from build123d import *

# Parameters (mm, degrees)
SKETCH_1_W          = 101.5
SKETCH_1_H          = 91.5
SKETCH_1_W_2        = 98.5
SKETCH_1_H_2        = 88.5
EXTRUDE_1_DEPTH     = 21
SKETCH_2_W          = 101.5
SKETCH_2_H          = 91.5
SKETCH_2_R          = 8.25
SKETCH_2_R_2        = 6
EXTRUDE_2_DEPTH     = 1.8
SKETCH_3_R          = 1.75
CUT_EXTRUDE_1_DEPTH = 139.25881527
SKETCH_4_R          = 1.75
CUT_EXTRUDE_2_DEPTH = 139.25881527
FILLET_1_R          = 9
FILLET_2_R          = 10
FILLET_3_R          = 4
FILLET_4_R          = 5
CUT_EXTRUDE_3_DEPTH = 1
CUT_EXTRUDE_4_REACH = 140.259
SKETCH_6_R          = 5.25


with BuildPart() as part:
    # 草图1 → 凸台-拉伸1 (new body)
    with BuildSketch(Plane(origin=(0, 0, 0), x_dir=(0, 0, -1), z_dir=(1, 0, 0))):
        with Locations((50.75, 45.75)):
            Rectangle(SKETCH_1_W, SKETCH_1_H)
        with Locations((50.75, 45.75)):
            Rectangle(SKETCH_1_W_2, SKETCH_1_H_2, mode=Mode.SUBTRACT)
    extrude(amount=EXTRUDE_1_DEPTH)

    # 草图2 → 凸台-拉伸2 (add)
    with BuildSketch(Plane.ZY):
        with Locations((-50.75, 45.75)):
            Rectangle(SKETCH_2_W, SKETCH_2_H)
        with Locations((-86.5, 76.5)):
            Circle(SKETCH_2_R, mode=Mode.SUBTRACT)
        with Locations((-50.75, 43.5)):
            Circle(SKETCH_2_R_2, mode=Mode.SUBTRACT)
    extrude(amount=EXTRUDE_2_DEPTH)

    # 草图3 → 切除-拉伸1 (cut, through all)
    with BuildSketch(Plane.XY):
        with Locations((11, 45.75)):
            Circle(SKETCH_3_R)
    extrude(amount=-CUT_EXTRUDE_1_DEPTH, mode=Mode.SUBTRACT)

    # 草图4 → 切除-拉伸2 (cut, through all)
    with BuildSketch(Plane(origin=(0, 91.5, 0), x_dir=(1, 0, 0), z_dir=(0, 1, 0))):
        with Locations(Location((11, 16.75, 0), (0, 0, 270))):
            Circle(SKETCH_4_R)
        with Locations(Location((11, 84.75, 0), (0, 0, 90))):
            Circle(SKETCH_4_R)
    extrude(amount=-CUT_EXTRUDE_2_DEPTH, mode=Mode.SUBTRACT)

    # 圆角1
    fillet_1_edges = [part.edges().sort_by_distance(p)[0] for p in [
        (10.5, 90, -100),
        (10.5, 90, -1.5),
    ]]
    fillet(fillet_1_edges, radius=FILLET_1_R)

    # 圆角2
    fillet_2_edges = [part.edges().sort_by_distance(p)[0] for p in [
        (9.6, 91.5, 0),
        (9.6, 91.5, -101.5),
    ]]
    fillet(fillet_2_edges, radius=FILLET_2_R)

    # 圆角3
    fillet_3_edges = [part.edges().sort_by_distance(p)[0] for p in [
        (10.5, 1.5, -1.5),
        (10.5, 1.5, -100),
    ]]
    fillet(fillet_3_edges, radius=FILLET_3_R)

    # 圆角4
    fillet_4_edges = [part.edges().sort_by_distance(p)[0] for p in [
        (9.6, 0, -101.5),
        (9.6, 0, 0),
    ]]
    fillet(fillet_4_edges, radius=FILLET_4_R)

    # 草图5 → 切除-拉伸3 (cut)
    with BuildSketch(Plane.ZY.offset(1.8)):
        with BuildLine():
            Line((-30.75, 43.5), (-20.75, 43.5))
            ThreePointArc((-20.75, 43.5), (-45.75, 68.5), (-70.75, 43.5))
            ThreePointArc((-70.75, 43.5), (-50.75, 63.5), (-30.75, 43.5))
        make_face()
    extrude(amount=-CUT_EXTRUDE_3_DEPTH, mode=Mode.SUBTRACT)

    # 草图6 → 切除-拉伸4 (cut, up to next)
    with BuildSketch(Plane.XY, mode=Mode.PRIVATE) as cut_extrude_4_sk1:
        with Locations((9, 74.75)):
            Circle(SKETCH_6_R)
    cut_extrude_4_tool1 = extrude(cut_extrude_4_sk1.sketch, amount=-CUT_EXTRUDE_4_REACH, mode=Mode.PRIVATE) & part.part
    add(cut_extrude_4_tool1.solids().sort_by_distance((9, 74.75, 0))[0], mode=Mode.SUBTRACT)


solid = part.part
Could you check a few things on this model? Use its own coordinates, in mm. A direction names the side the tool comes from. Give positions to 0.01 mm unless a question says otherwise; leave off trailing zeros. Write each loop counter-clockwise with the first axis right and the second up, starting at its lowest first coordinate (ties: lowest second). Pieces come first, ordered by that corner, then holes. Notation, with made-up numbers: (2.5, -33) -> (29.5, -33) arc R23 cw to (29.5, 5) -> close; hole circle Ø4 at (-6.5, 36). An arc over 180 degrees is marked (long way). Answer as CSV lines item,"result". Start each with the question number.
(1) Which directions (+Z, -Z, +X, -X, +Y, -Y) give clear straight access to the entire face, cutting with the end or side of a thin tool? Please do faces 1 (the face through (-0.8, 57.9, -36.6)), 2 (the face through (10.647, 87.294, -97.434)), 3 (the face through (12.18, 0.76, -18.04)).
(2) Please list where these lines run through material, in increasing order: line 1 (Y direction, x = 15.5, z = -54.5); line 2 (Z direction, x = 6.5, y = 41.5); line 3 (Y direction, x = -1.2, z = -86.5).
(3) If we section it at A-A, the plane z = -16.75: Write out the boundary of the cut face in (x, y), and give its area (3 significant figures).
(4) If we section it at C-C, the plane y = 45.75: Give the number of separate pieces and of enclosed holes in the cut face, and give its area (3 significant figures).
(5) I'm going to push flat-ended pins straight in: pin 1 Ø3 at (x, z) = (11, -84.75) entering from +Y; pin 2 Ø4 at (y, z) = (44.5, -82.5) entering from +X. Where does each tip first touch, or does it pass through?
(6) If we section it at B-B, the plane x = 18.25: Write out the boundary of the cut face in (y, z).
(7) If we mould it in two halves opening along Y, with no side actions, what happens to faces 4 (the face through (10, 43, -1.5)), 5 (the face through (-1.307, 68.494, -45.2)), 6 (the face through (12.18, 90.76, -18.04)), 7 (the face through (9.76, 88.65, -98.49))? For each: +Y half, -Y half, draft (parallel to the pull), parting line (faces both ways), or undercut.
(8) If we section it at D-D, the plane y = 33.5: Write out the boundary of the cut face in (x, z), and give its area (3 significant figures).
Answer list:
1,face 1,"-X"
1,face 2,"+X"
1,face 3,"+Y, -Y"
2,line 1,"0 to 1.5, 90 to 91.5"
2,line 2,"-101.5 to -100, -1.5 to 0"
2,line 3,"0 to 68.25, 84.75 to 91.5"
3,outline,"(-1.8, 0) -> (9.25, 0) -> (9.25, 1.5) -> (0, 1.5) -> (0, 90) -> (9.25, 90) -> (9.25, 91.5) -> (-1.8, 91.5) -> close; (12.75, 0) -> (21, 0) -> (21, 1.5) -> (12.75, 1.5) -> close; (12.75, 90) -> (21, 90) -> (21, 91.5) -> (12.75, 91.5) -> close"
3,area,"217 mm^2"
4,separate pieces,"4"
4,enclosed holes,"0"
4,area,"205 mm^2"
5,pin 1,"through"
5,pin 2,"x = 0"
6,outline,"(0, -96.5) arc R5 ccw to (5, -101.5) -> (81.5, -101.5) arc R10 ccw to (91.5, -91.5) -> (91.5, -10) arc R10 ccw to (81.5, 0) -> (5, 0) arc R5 ccw to (0, -5) -> close; hole (1.5, -96) arc R4 ccw to (5.5, -100) -> (81, -100) arc R9 ccw to (90, -91) -> (90, -10.5) arc R9 ccw to (81, -1.5) -> (5.5, -1.5) arc R4 ccw to (1.5, -5.5) -> close"
7,face 4,"undercut"
7,face 5,"undercut"
7,face 6,"draft"
7,face 7,"+Y half"
8,outline,"(-1.8, -101.5) -> (21, -101.5) -> (21, -100) -> (0, -100) -> (0, -1.5) -> (21, -1.5) -> (21, 0) -> (-1.8, 0) -> close"
8,area,"246 mm^2"
